Can you work these out from the model? Positions are in its coordinate system, mm. Face numbers are marked on the shaded views. A direction names the side the tool comes from. Coordinates: 2 decimals unless noted, no trailing zeros. Loops run counter-clockwise (first coordinate to the right, second up) from the corner with the lowest first, then second, coordinate; pieces in that order, holes last. Notation, with made-up numbers: M -12,-34 L 46,-34 A24 cw 46,3 Z; hole C 4,35.25 d6. An arc over 180 degrees is marked long. Answer as a JSON object with one key per item and string values. Group by question number.
Item 1: Which directions (+Z, -Z, +X, -X, +Y, -Y) give clear straight access to the entire face, cutting with the end or side of a thin tool? Please do the marked faces 1, 2 and 3.
Item 2: Suppose I cut it at B-B (x = 0). Write out the boundary of the cut face in (y, z).
Item 3: If I drill on line 1 (Z direction, x = -41, y = 9); line 2 (Y direction, x = 0, z = 61); line 3 (Z direction, x = 47.5, y = 4.5), over which ranges is the centre line in solid material (lowest first)?
Item 4: Suppose I cut it at D-D (z = -45.5). Write out the boundary of the cut face in (x, y).
Item 5: Suppose I cut it at A-A (z = 60). Write out the boundary of the cut face in (x, y).
Item 6: I'm going to push flat-ended pins straight in: pin 1 Ø8 at (x, y) = (0, 77) entering from -Z; pin 2 Ø22 at (x, y) = (0, 77) entering from -Z; pin 3 Ø1 at (x, z) = (1, -52) entering from +Y. Where does each tip first touch, or does it pass through?
Item 7: Suppose I cut it at C-C (x = 46.5). Write out the boundary of the cut face in (y, z), then the cut area to 3 significant figures.
```python
from build123d import *

# Parameters (mm, degrees)
SKETCH1_W                = 140
SKETCH1_H                = 140
SKETCH1_W_2              = 100
SKETCH1_H_2              = 100
BOSS_EXTRUDE1_DEPTH      = 10
BOSS_EXTRUDE2_DEPTH      = 3
BOSS_EXTRUDE2_DEPTH_BACK = 10
SKETCH4_R                = 8.55
CUT_EXTRUDE2_DEPTH       = 6
SKETCH5_R                = 3.5
CUT_EXTRUDE3_DEPTH       = 178.803262062
FILLET1_R                = 5
CUT_EXTRUDE4_START       = 5
SKETCH6_W                = 40
SKETCH6_H                = 55
CUT_EXTRUDE4_DEPTH       = 133.20422734
SKETCH6_3_W              = 40
SKETCH6_3_H              = 55
BOSS_EXTRUDE4_DEPTH      = 5


with BuildPart() as part:
    # Sketch1 → Boss-Extrude1 (new body)
    with BuildSketch(Plane(origin=(0, 0, 0), x_dir=(1, 0, 0), z_dir=(0, 1, 0))):
        Rectangle(SKETCH1_W, SKETCH1_H)
        Rectangle(SKETCH1_W_2, SKETCH1_H_2, mode=Mode.SUBTRACT)
    extrude(amount=BOSS_EXTRUDE1_DEPTH)

    # Sketch2 → Boss-Extrude2 (add, two sides: drawn at the far end of the back side and taken through both)
    with BuildSketch(Plane(origin=(0, 0, 60), x_dir=(-1, 0, 0), z_dir=(0, 0, -1)).offset(-BOSS_EXTRUDE2_DEPTH_BACK)):
        with BuildLine():
            Line((55, 10), (-55, 10))
            Line((-55, 10), (-13.187649977, 87.147439268))
            ThreePointArc((-13.187649977, 87.147439268), (0, 95), (13.187649977, 87.147439268))
            Line((13.187649977, 87.147439268), (55, 10))
        make_face()
    extrude(amount=BOSS_EXTRUDE2_DEPTH + BOSS_EXTRUDE2_DEPTH_BACK)

    # Sketch4 → Cut-Extrude2 (cut)
    with BuildSketch(Plane(origin=(0, 0, 57), x_dir=(-1, 0, 0), z_dir=(0, 0, -1))):
        with Locations((0, 77)):
            Circle(SKETCH4_R)
    extrude(amount=-CUT_EXTRUDE2_DEPTH, mode=Mode.SUBTRACT)

    # Sketch5 → Cut-Extrude3 (cut, through all)
    with BuildSketch(Plane(origin=(0, 0, 63), x_dir=(-1, 0, 0), z_dir=(0, 0, -1))):
        with Locations((0, 77)):
            Circle(SKETCH5_R)
    extrude(amount=-CUT_EXTRUDE3_DEPTH, mode=Mode.SUBTRACT)

    # Fillet1
    fillet1_edges = [part.edges().sort_by_distance(p)[0] for p in [
        (70, 5, 70),
        (-70, 5, 70),
        (-70, 5, -70),
        (70, 5, -70),
    ]]
    fillet(fillet1_edges, radius=FILLET1_R)

    # Sketch6 → Cut-Extrude4 (cut, through all)
    with BuildSketch(Plane(origin=(0, 0, 0), x_dir=(1, 0, 0), z_dir=(0, 1, 0)).offset(CUT_EXTRUDE4_START)):
        with Locations((50, -42.5)):
            Rectangle(SKETCH6_W, SKETCH6_H)
    extrude(amount=CUT_EXTRUDE4_DEPTH, mode=Mode.SUBTRACT)

    # Sketch6<3> → Boss-Extrude4 (add)
    with BuildSketch(Plane(origin=(0, 0, 0), x_dir=(1, 0, 0), z_dir=(0, 1, 0))):
        with Locations((50, -42.5)):
            Rectangle(SKETCH6_3_W, SKETCH6_3_H)
    extrude(amount=BOSS_EXTRUDE4_DEPTH)


solid = part.part
```
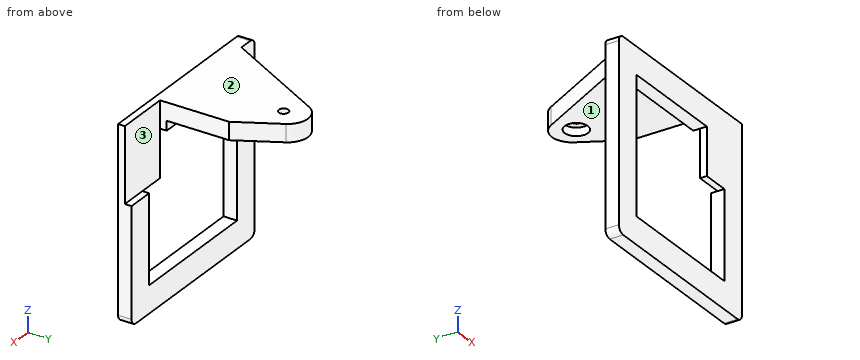
From the geometry:
{
 "1": {"face 1": "-Z, +X, -X, +Y", "face 2": "+Z, +X, -X, +Y, -Y", "face 3": "+Z, +X, +Y"},
 "2": {"outline": "M 0,-70 L 10,-70 L 10,-50 L 0,-50 Z; M 0,50 L 10,50 L 10,57 L 68.45,57 L 68.45,63 L 73.5,63 L 73.5,70 L 0,70 Z; M 80.5,63 L 85.55,63 L 85.55,57 L 95,57 L 95,70 L 80.5,70 Z"},
 "3": {"line 1": "-70 to -50, 50 to 70", "line 2": "0 to 68.45, 85.55 to 95", "line 3": "-70 to -50, 15 to 70"},
 "4": {"outline": "M -70,0 L -50,0 L -50,10 L -70,10 Z; M 50,0 L 70,0 L 70,10 L 50,10 Z"},
 "5": {"outline": "M -70,0 L 70,0 L 70,5 L 30,5 L 30,56.13 L 13.19,87.15 A15 ccw -13.19,87.15 L -55,10 L -70,10 Z; hole C 0,77 d17.1"},
 "6": {"pin 1": "z = 63", "pin 2": "z = 57", "pin 3": "y = 10"},
 "7": {"outline": "M 0,-70 L 10,-70 L 10,-50 L 0,-50 Z; M 0,15 L 5,15 L 5,70 L 0,70 Z", "area": "475 mm2"}
}
